Job drawing, mm, ordinate dimensions from the low corner. One solid piece. A direction names the side the tool comes from. Give positions to 0.01 mm unless a question says otherwise; leave off trailing zeros. Loops run counter-clockwise (first coordinate to the right, second up) from the corner with the lowest first, then second, coordinate; pieces in that order, holes last. Notation, with made-up numbers: M -37,-39 L 15,-39 A21 cw 15,-27 Z; hole C 67.5,77.5 d2. An arc over 180 degrees is marked long. Put each result on its own line as item: value.
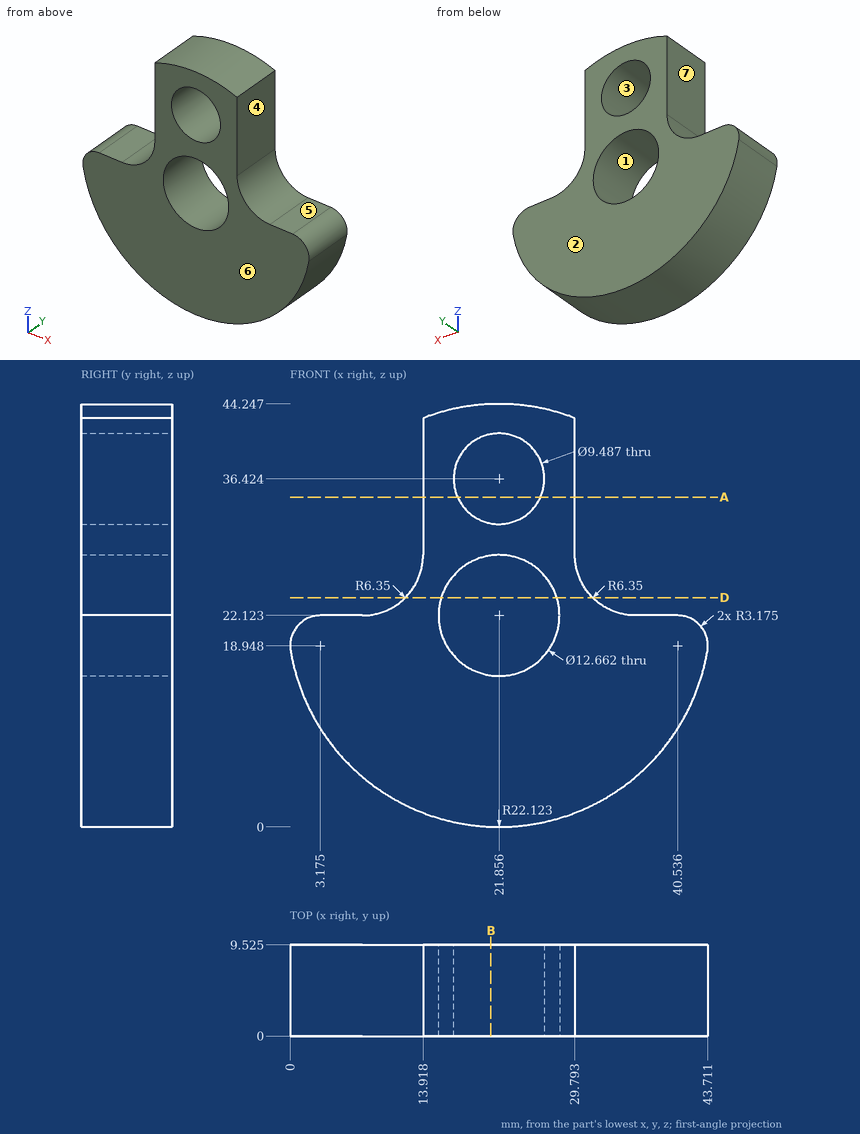
Q1. Probe line 1 (Z direction, x = 18.5, y = 4.25) (1 decimal); line 2 (X direction, y = 0.5, z = 36.5); line 3 (X direction, y = 0.5, z = 31.5). List the from-to ranges inside material, lowest first. Write a range as from..to.
Here are the results:
line 1: 0.3..16.8, 27.5..33.1, 39.8..44
line 2: 13.92..17.11, 26.6..29.79
line 3: 13.92..29.79
Q2. Slice it at A-A (z = 34.5). List the corners of the cut face in (x, y) (1 decimal).
Here are the results:
outline: M 13.9,0 L 17.5,0 L 17.5,9.5 L 13.9,9.5 Z; M 26.2,0 L 29.8,0 L 29.8,9.5 L 26.2,9.5 Z
Q3. Mould opens along X. For the marked faces 1, 2, 3 and 4 say: pulls with the +X half, pulls with the -X half, needs draft (parallel to the pull), parting line crosses it, or undercut.
Here are the results:
face 1: undercut
face 2: needs draft
face 3: undercut
face 4: pulls with the +X half
Q4. Slice it at D-D (z = 24). List the corners of the cut face in (x, y) (1 decimal).
Here are the results:
outline: M 12.1,0 L 15.8,0 L 15.8,9.5 L 12.1,9.5 Z; M 27.9,0 L 31.6,0 L 31.6,9.5 L 27.9,9.5 Z
Q5. Drop flat-ended pins along their axis: pin 1 Ø1 at (y, z) = (3, 13) entering from +X; pin 2 Ø1.3 at (x, y) = (37.5, 7) entering from +Z; pin 3 Ø5 at (y, z) = (6.5, 32) entering from -X. Give the stop position or say it passes through.
Here are the results:
pin 1: x = 42.23
pin 2: z = 22.12
pin 3: x = 13.92
Q6. Tool access for the marked faces 5, 6 and 7: list every direction of +Z, -Z, +X, -X, +Y, -Y with a clear straight run to the whole face (end or side of a thin tool).
Here are the results:
face 5: +Z, +X, +Y, -Y
face 6: +Z, -Z, +X, -X, -Y
face 7: +Z, -X, +Y, -Y
Q7. Slice it at B-B (x = 21). State how many separate pieces and enclosed holes the cut face has, and give its area (3 significant figures).
Here are the results:
separate pieces: 3
enclosed holes: 0
area: 213 mm²
